Input: part model. Units: mm. Frame: model coordinates. Face numbers are marked on the shaded views. Give positions to 0.01 mm unless a question says otherwise; leave off trailing zeros. Loops run counter-clockwise (first coordinate to the right, second up) from the corner with the lowest first, then second, coordinate; pieces in that order, holes last. Notation, with made-up numbers: M 57,37.5 L 82,37.5 A23 cw 82,54.5 Z; hole C -4,-26.75 d6. An arc over 180 degrees is marked long. One line per item, written item: value. Start each with the question number.
(1) Pull-direction query (Z, two-part tool) for the marked faces 1, 2 and 3; classes: released by +Z, released by -Z, zero draft, split by the parting line, or undercut.
(2) Section B-B on y = 0. Output: boundary loops of the cut face in (x, z), plus the area to 3 significant figures.
(3) Pin query (flat end, axial travel): P1, Ø6, axis at x = 4.5, z = -51.5, coming from the -Y side (3 decimals); P2, Ø10, axis at y = -77.5, z = -479.5, coming from the -X side; P3, Ø1, axis at x = -63, y = 289.5, coming from the -Z side. Return the tip coordinate at first contact, or that it passes through.
(4) Ray query, line 1 along Z through (x, y) = (44.5, 178); line 2 along Z through (x, y) = (-6, 260.5); line 3 along Y through (x, z) = (129.5, -672). Return the intervals inside material, ascending. Write a range as from..to.
(5) Section A-A on z = 0. Output: boundary loops of the cut face in (x, y), plus the area to 3 significant figures.
(6) Section D-D on y = 203.5. Output: boundary loops of the cut face in (x, z), plus the area to 3 significant figures.
```python
from build123d import *

# Parameters (mm, degrees)
SKETCH2_R           = 75
SKETCH3_R           = 100
BOSS_EXTRUDE1_DEPTH = 62.5
CHAMFER1_SIZE       = 12.5


with BuildPart() as part:
    # Sweep1: sweep along a path in Sketch1
    with BuildLine(Plane(origin=(0, 0, 0), x_dir=(0, 0, -1), z_dir=(1, 0, 0))) as sweep1_path:
        Line((0, 695.970875), (0, 0))
        Line((0, 0), (737.5, 0))
    # Sketch2 → Sweep1 (sweep)
    with BuildSketch(Plane(origin=(0, 695.970875, 0), x_dir=(1, 0, 0), z_dir=(0, 1, 0))):
        Circle(SKETCH2_R)
    sweep(path=sweep1_path.line, transition=Transition.RIGHT)

    # Sketch3 → Boss-Extrude1 (add)
    with BuildSketch(Plane(origin=(0, 695.970875, 0), x_dir=(1, 0, 0), z_dir=(0, 1, 0))):
        Circle(SKETCH3_R)
    extrude(amount=-BOSS_EXTRUDE1_DEPTH)

    # Sketch4 → Revolve1 (revolve)
    with BuildSketch(Plane(origin=(0, 0, 0), x_dir=(0, 0, -1), z_dir=(1, 0, 0))):
        Polygon((137.5, 75), (137.5, 187.5), (187.5, 187.5), (187.5, 156.25), (687.5, 156.25), (687.5, 187.5), (737.5, 187.5), (737.5, 75), align=None)
    revolve(axis=Axis((0, 0, -737.5), (0, 0, 1)))

    # Chamfer1
    chamfer1_edges = [part.edges().sort_by_distance(p)[0] for p in [
        (-75, 0, -137.5),
        (0, -187.5, -137.5),
        (0, -156.25, -187.5),
        (0, -156.25, -687.5),
        (0, -187.5, -737.5),
    ]]
    chamfer(chamfer1_edges, length=CHAMFER1_SIZE)


solid = part.part
```
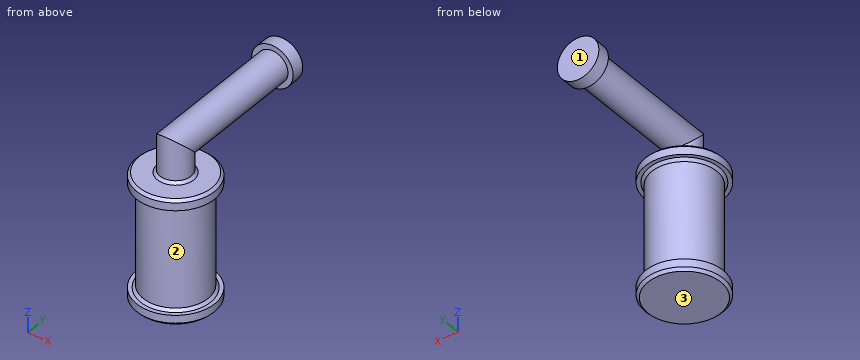
Output values:
1. face 1: zero draft
1. face 2: undercut
1. face 3: released by -Z
2. outline: M -187.5,-725 L -175,-737.5 L 175,-737.5 L 187.5,-725 L 187.5,-687.5 L 168.75,-687.5 L 156.25,-675 L 156.25,-200 L 168.75,-187.5 L 187.5,-187.5 L 187.5,-150 L 175,-137.5 L 87.5,-137.5 L 75,-125 L 75,0 A75 ccw -75,0 L -75,-125 L -87.5,-137.5 L -175,-137.5 L -187.5,-150 L -187.5,-187.5 L -168.75,-187.5 L -156.25,-200 L -156.25,-675 L -168.75,-687.5 L -187.5,-687.5 Z
2. area: 223,000 mm²
3. P1: stops at y = -74.985
3. P2: stops at x = -138.41
3. P3: stops at z = -41.46
4. line 1: z = -729.02..-687.5, -187.5..-145.98, -60.37..60.37
4. line 2: z = -74.76..74.76
4. line 3: y = -87.43..87.43
5. outline: M -100,633.47 L -75,633.47 L -75,0 A75 ccw 75,0 L 75,633.47 L 100,633.47 L 100,695.97 L -100,695.97 Z
5. area: 116,000 mm²
6. outline: C 0,0 d150
6. area: 17,700 mm²
